Input: dimensioned drawing with shaded views. Units: mm. Origin: part minimum x, y, z. A direction names the side the tool comes from. Give positions to 0.01 mm unless a question says otherwise; leave off trailing zeros. Loops run counter-clockwise (first coordinate to the right, second up) from the corner with the lowest first, then second, coordinate; pieces in that order, holes last. Notation, with made-up numbers: (-27.5, 47) -> (1.5, 47) arc R15 cw to (1.5, 55) -> close; hole circle Ø10 at (-7, 59.5). An arc over 180 degrees is marked (long way). Answer as a JSON object with one key per item and string values.
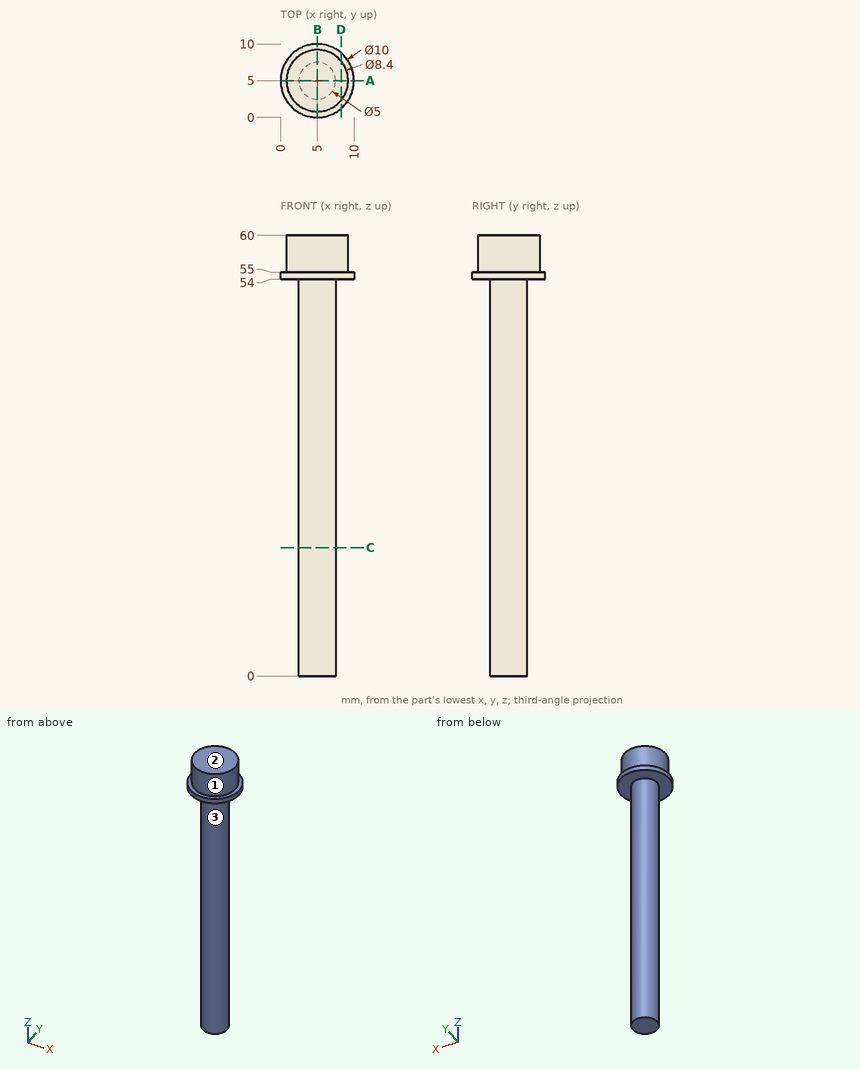
Q1. Pin query (flat end, axial travel): pin 1 (1 mm diameter, centred on x = 2.5, z = 40, fed in from +Y); pin 2 (1.5 mm diameter, centred on y = 7.5, z = 17.5, fed in from +X); pin 3 (1.5 mm diameter, centred on x = 8, z = 53.5, fed in from -Y). Return the tip coordinate at first contact, or that it passes through.
Evaluation:
{"pin 1": "stops at y = 6.5", "pin 2": "stops at x = 6.79", "pin 3": "stops at y = 0.64"}
Q2. Section D-D, the plane x = 8.25. Return the cut outline in (y, z), then the cut area to 3 significant figures.
Evaluation:
{"outline": "(1.2, 54) -> (8.8, 54) -> (8.8, 55) -> (7.66, 55) -> (7.66, 60) -> (2.34, 60) -> (2.34, 55) -> (1.2, 55) -> close", "area": "34.2 mm2"}
Q3. Ray query, line 1 along Z through (x, y) = (8.25, 1.5); line 2 along Z through (x, y) = (8.25, 7.5); line 3 along Y through (x, z) = (5, 52). Return the intervals inside material, ascending.
Evaluation:
{"line 1": "z = 54 to 55", "line 2": "z = 54 to 60", "line 3": "y = 2.5 to 7.5"}
Q4. Access query for the marked faces 1, 2 and 3. Directions: +Z, -Z, +X, -X, +Y, -Y. A direction counts if a zero-diameter tool reaches every point of the face in a straight line with its end or side. Return the directions, or none.
Evaluation:
{"face 1": "+Z", "face 2": "+Z, +X, -X, +Y, -Y", "face 3": "-Z"}
Q5. Section A-A, the plane y = 5. Return the cut outline in (x, z), then the cut area to 3 significant figures.
Evaluation:
{"outline": "(0, 54) -> (2.5, 54) -> (2.5, 0) -> (7.5, 0) -> (7.5, 54) -> (10, 54) -> (10, 55) -> (9.2, 55) -> (9.2, 60) -> (0.8, 60) -> (0.8, 55) -> (0, 55) -> close", "area": "322 mm2"}
Q6. Section C-C, the plane z = 17.5. Return the cut outline in (x, y), then the cut area to 3 significant figures.
Evaluation:
{"outline": "circle Ø5 at (5, 5)", "area": "19.6 mm2"}
